Verification items for the finished model (mm, model axes). Round coordinates to 2 decimals unless told otherwise and drop trailing zeros. Write each loop counter-clockwise with the first axis right and the second up, starting at its lowest first coordinate (ties: lowest second). Pieces come first, ordered by that corner, then holes. Notation, with made-up numbers: M -27,-32.75 L 14,-32.75 A26 ccw 14,-7.75 Z; hole C -10.5,43 d1. An arc over 180 degrees is marked long. One line per question, with ' | ' between items.
from build123d import *

# Parameters (mm, degrees)
SKETCH1_W                = 158.75
SKETCH1_H                = 263.525
BOSS_EXTRUDE1_DEPTH      = 3
SKETCH5_R                = 11.1125
CUT_EXTRUDE1_DEPTH       = 154.853004622
M3_CLEARANCE_HOLE1_D     = 3.2
M3_CLEARANCE_HOLE1_DEPTH = 3
M5_CLEARANCE_HOLE2_D     = 5.3
M5_CLEARANCE_HOLE2_DEPTH = 3
FILLET1_R                = 6.35


with BuildPart() as part:
    # Sketch1 → Boss-Extrude1 (new body)
    with BuildSketch(Plane(origin=(0, 0, 0), x_dir=(1, 0, 0), z_dir=(0, 1, 0))):
        Rectangle(SKETCH1_W, SKETCH1_H)
    extrude(amount=BOSS_EXTRUDE1_DEPTH)

    # Sketch5 → Cut-Extrude1 (cut, through all)
    with BuildSketch(Plane(origin=(0, 3, 0), x_dir=(1, 0, 0), z_dir=(0, 1, 0))):
        with Locations(Location((0, 0, 0), (0, 0, 270))):
            Circle(SKETCH5_R)
    extrude(amount=-CUT_EXTRUDE1_DEPTH, mode=Mode.SUBTRACT)

    # M3 Clearance Hole1
    with Locations(Plane(origin=(0, 3, 0), x_dir=(1, 0, 0), z_dir=(0, 1, 0))):
        with Locations((0, 0), (15.5, 15.5), (-15.5, -15.5), (-15.5, 15.5), (15.5, -15.5)):
            Hole(M3_CLEARANCE_HOLE1_D / 2, depth=M3_CLEARANCE_HOLE1_DEPTH)

    # M5 Clearance Hole2
    with Locations(Plane(origin=(0, 3, 0), x_dir=(1, 0, 0), z_dir=(0, 1, 0))):
        with Locations((0, 0), (71.4375, 123.825), (-71.4375, -123.825), (-71.4375, 123.825), (71.4375, -123.825), (-71.4375, 0), (71.4375, 0)):
            Hole(M5_CLEARANCE_HOLE2_D / 2, depth=M5_CLEARANCE_HOLE2_DEPTH)

    # Fillet1
    fillet1_edges = [part.edges().sort_by_distance(p)[0] for p in [
        (79.375, 1.5, 131.7625),
        (-79.375, 1.5, 131.7625),
        (-79.375, 1.5, -131.7625),
        (79.375, 1.5, -131.7625),
    ]]
    fillet(fillet1_edges, radius=FILLET1_R)


solid = part.part
1. Thickness scan on line 1 (X direction, y = 1.5, z = 15.5) (3 decimals); line 2 (Z direction, x = 15.5, y = 0.6); line 3 (X direction, y = 1.9, z = 6) (3 decimals). Record the ranges inside material, lowest first.
Results:
line 1: x = -79.375 to -17.1, -13.9 to 13.9, 17.1 to 79.375 | line 2: z = -131.76 to -17.1, -13.9 to 13.9, 17.1 to 131.76 | line 3: x = -79.375 to -9.353, 9.353 to 79.375
2. Mould release check, pull along X, two halves, no side actions. Record for faces 1 (the face through (-77.564, 1.521, 129.853)), 2 (the face through (71.8, 1.5, 121.2)), 3 (the face through (77.47, 1.52, -129.95)), 4 (the face through (-71.093, 1.479, 121.198)): pulls with the +X half, pulls with the -X half, needs draft (parallel to the pull), parting line crosses it, or undercut.
Results:
face 1: pulls with the -X half | face 2: undercut | face 3: pulls with the +X half | face 4: undercut
3. Section check B-B, the plane z = 0. Record the cut outline in (x, y) (1 decimal), then the cut area to 3 significant figures.
Results:
outline: M -79.4,0 L -74.1,0 L -74.1,3 L -79.4,3 Z; M -68.8,0 L -11.1,0 L -11.1,3 L -68.8,3 Z; M 11.1,0 L 68.8,0 L 68.8,3 L 11.1,3 Z; M 74.1,0 L 79.4,0 L 79.4,3 L 74.1,3 Z | area: 378 mm2
4. Section check A-A, the plane x = 0. Record the cut outline in (y, z).
Results:
outline: M 0,-131.76 L 3,-131.76 L 3,-11.11 L 0,-11.11 Z; M 0,11.11 L 3,11.11 L 3,131.76 L 0,131.76 Z
5. Go/stop test with a flat-tipped pin: P1, Ø7, axis at x = -71.44, z = 0, coming from the +Y side. Record where the tip stops, or that it passes through.
Results:
P1: stops at y = 3
